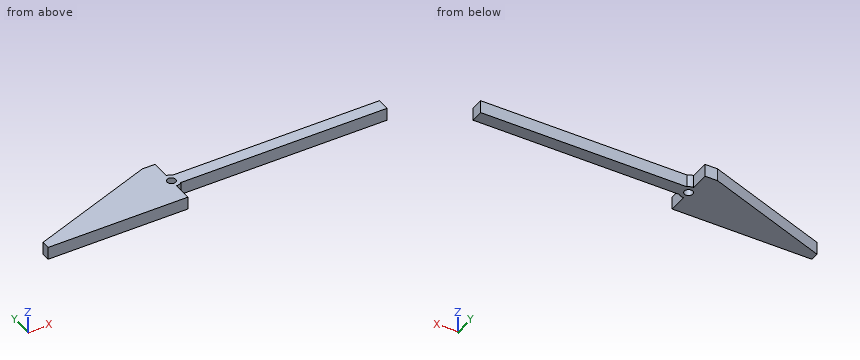
from build123d import *

# Parameters (mm, degrees)
SKETCH_1_R      = 1
EXTRUDE_1_DEPTH = 3


with BuildPart() as part:
    # Эскиз1 → Бобышка-Вытянуть1 (new body)
    with BuildSketch(Plane.XY):
        with BuildLine():
            Line((0, 0), (0, 2))
            Line((0, 2), (30, 12.919107028))
            Line((30, 12.919107028), (33, 12.919107028))
            Line((33, 12.919107028), (33, 8.459553514))
            ThreePointArc((33, 8.459553514), (33.707106781, 8.330382207), (34.322875656, 7.959553514))
            Line((34.322875656, 7.959553514), (83, 7.959553514))
            Line((83, 7.959553514), (83, 4.959553514))
            Line((83, 4.959553514), (34.322875656, 4.959553514))
            ThreePointArc((34.322875656, 4.959553514), (33.707106781, 4.588724821), (33, 4.459553514))
            Line((33, 4.459553514), (33, 0))
            Line((33, 0), (0, 0))
        make_face()
        with Locations((33, 6.459553514)):
            Circle(SKETCH_1_R, mode=Mode.SUBTRACT)
    extrude(amount=EXTRUDE_1_DEPTH)


solid = part.part
Check sheet for the modelled part. Datum: model origin and axes. Units: mm. Give positions to 0.01 mm unless a question says otherwise; leave off trailing zeros. Write each loop counter-clockwise with the first axis right and the second up, starting at its lowest first coordinate (ties: lowest second). Pieces come first, ordered by that corner, then holes. Notation, with made-up numbers: (26, 13.5) -> (65, 13.5) arc R26 cw to (65, 48.5) -> close; hole circle Ø1 at (-5, -38). An arc over 180 degrees is marked (long way). Write item = value, one per line.
Item 1: Scan lines: probe 1 along X at (y, z) = (1, 0.2); probe 2 along Y at (x, z) = (44.5, 1.6); probe 3 along Y at (x, z) = (6, 0.2). Record each from-to range of solid material in increasing order. Write a range as from..to.
Output:
probe_1 = 0..33
probe_2 = 4.96..7.96
probe_3 = 0..4.18
Item 2: Sectioned sample at B-B on x = 47.5. Record the boundary of the cut face in (y, z).
Output:
outline = (4.96, 0) -> (7.96, 0) -> (7.96, 3) -> (4.96, 3) -> close
Item 3: Gauge pin test, flat ends, axial feed: pin 1 (1.5 mm diameter, centred on y = 4.5, z = 2, fed in from +X); pin 2 (1.5 mm diameter, centred on y = 1.5, z = 1, fed in from +X). Record the tip position at first contact, or that the pin passes through.
Output:
pin_1 = 83
pin_2 = 33
Item 4: Sectioned sample at C-C on y = 9.25. Record the boundary of the cut face in (x, z).
Output:
outline = (19.92, 0) -> (33, 0) -> (33, 3) -> (19.92, 3) -> close
Item 5: Sectioned sample at A-A on z = 0.6. Record the boundary of the cut face in (x, y), and give its area (3 significant figures).
Output:
outline = (0, 0) -> (33, 0) -> (33, 4.46) arc R2 ccw to (34.32, 4.96) -> (83, 4.96) -> (83, 7.96) -> (34.32, 7.96) arc R2 ccw to (33, 8.46) -> (33, 12.92) -> (30, 12.92) -> (0, 2) -> close; hole circle Ø2 at (33, 6.46)
area = 410 mm^2
